For this review, take the finished solid that the model builds, in its own axes (mm). Coordinates: 2 decimals unless noted, no trailing zeros. Order: outer loops, then holes, each group sorted by start corner. A loop starts at its lowest first (then second) coordinate and runs counter-clockwise, first axis right, second up. Notation, with made-up numbers: (48, 82) -> (95, 82) arc R24 cw to (95, 102) -> close; hole circle Ø7 at (15, 61). An arc over 180 degrees is marked (long way). Return JSON: item names as keys, results as strings. Group by question number.
Item 1: Draft analysis for pull direction Z (two halves, no side actions). For faces 1 (the cylindrical face through (-8.42, 1.288, -9.396)), 2 (the flat face through (-9.144, 1, 0)), 3 (the cylindrical face through (4.303, 1.288, 7.077)), state which applies: +Z half, -Z half, draft (parallel to the pull), parting line (faces both ways), or undercut.
Item 2: Take a section at A-A (x = -4.25). Write out the cut boundary in (y, z), then the cut area to 3 significant figures.
Item 3: For line 1 along Z through (x, y) = (-4.75, 1.45); line 2 along X through (y, z) = (0.1, 5.75); line 3 along X through (y, z) = (1.2, -4.5), list the stretches that pass through material, from the lowest coordinate up.
Item 4: Take a section at C-C (z = 6). Write out the cut boundary in (x, y).
Item 5: Insertion check: pin 1 (4 mm diameter, centred on x = 4.62, z = -5.64, fed in from -Y). The pin has a flat end and moves straight along its axis. Give the tip position at first contact, or say it passes through.
Item 6: Take a section at B-B (y = 0.5). Write out the cut boundary in (x, z), then the cut area to 3 significant figures.
```python
from build123d import *

# Parameters (mm, degrees)
SKETCH1_W           = 18.288
SKETCH1_H           = 20.32
BOSS_EXTRUDE1_DEPTH = 2.54
SKETCH2_R           = 1.4732
CUT_EXTRUDE1_DEPTH  = 3.54
FILLET1_R           = 2.54


with BuildPart() as part:
    # Sketch1 → Boss-Extrude1 (new body)
    with BuildSketch(Plane(origin=(0, 0, 0), x_dir=(1, 0, 0), z_dir=(0, 1, 0))):
        Rectangle(SKETCH1_W, SKETCH1_H)
    extrude(amount=BOSS_EXTRUDE1_DEPTH)

    # Sketch2 → Cut-Extrude1 (cut, through all)
    with BuildSketch(Plane(origin=(0, 2.54, 0), x_dir=(1, 0, 0), z_dir=(0, 1, 0))):
        with Locations((-4.6228, 5.6388)):
            Circle(SKETCH2_R)
        with Locations((-4.6228, -5.6388)):
            Circle(SKETCH2_R)
        with Locations((4.6228, -5.6388)):
            Circle(SKETCH2_R)
        with Locations((4.6228, 5.6388)):
            Circle(SKETCH2_R)
    extrude(amount=-CUT_EXTRUDE1_DEPTH, mode=Mode.SUBTRACT)

    # Fillet1
    fillet1_edges = [part.edges().sort_by_distance(p)[0] for p in [
        (9.144, 1.27, 10.16),
        (-9.144, 1.27, 10.16),
        (-9.144, 1.27, -10.16),
        (9.144, 1.27, -10.16),
    ]]
    fillet(fillet1_edges, radius=FILLET1_R)


solid = part.part
```
Findings below:
{
 "1": {"face 1": "-Z half", "face 2": "draft", "face 3": "undercut"},
 "2": {"outline": "(0, -10.16) -> (2.54, -10.16) -> (2.54, -7.06) -> (0, -7.06) -> close; (0, -4.21) -> (2.54, -4.21) -> (2.54, 4.21) -> (0, 4.21) -> close; (0, 7.06) -> (2.54, 7.06) -> (2.54, 10.16) -> (0, 10.16) -> close", "area": "37.1 mm2"},
 "3": {"line 1": "z = -10.16 to -7.11, -4.17 to 4.17, 7.11 to 10.16", "line 2": "x = -9.14 to -6.09, -3.15 to 3.15, 6.09 to 9.14", "line 3": "x = -9.14 to -5.56, -3.69 to 3.69, 5.56 to 9.14"},
 "4": {"outline": "(-9.14, 0) -> (-6.05, 0) -> (-6.05, 2.54) -> (-9.14, 2.54) -> close; (-3.19, 0) -> (3.19, 0) -> (3.19, 2.54) -> (-3.19, 2.54) -> close; (6.05, 0) -> (9.14, 0) -> (9.14, 2.54) -> (6.05, 2.54) -> close"},
 "5": {"pin 1": "stops at y = 0"},
 "6": {"outline": "(-9.14, -7.62) arc R2.54 ccw to (-6.6, -10.16) -> (6.6, -10.16) arc R2.54 ccw to (9.14, -7.62) -> (9.14, 7.62) arc R2.54 ccw to (6.6, 10.16) -> (-6.6, 10.16) arc R2.54 ccw to (-9.14, 7.62) -> close; hole circle Ø2.95 at (-4.62, -5.64); hole circle Ø2.95 at (-4.62, 5.64); hole circle Ø2.95 at (4.62, -5.64); hole circle Ø2.95 at (4.62, 5.64)", "area": "339 mm2"}
}
